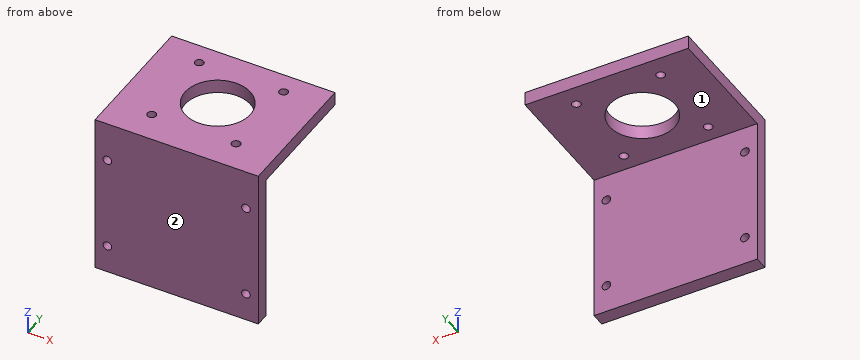
from build123d import *

# Parameters (mm, degrees)
EXTRUDE_1_DEPTH = 60
HOLE_WIZARD_2_D = 24
HOLE_WIZARD_3_D = 3.2
HOLE_WIZARD_4_D = 3.2


with BuildPart() as part:
    # 草图1 → 凸台-拉伸1 (new body)
    with BuildSketch(Plane(origin=(0, 0, 0), x_dir=(0, 0, -1), z_dir=(1, 0, 0))):
        Polygon((0, 0), (0, 50), (5, 50), (5, 5), (60, 5), (60, 0), align=None)
    extrude(amount=EXTRUDE_1_DEPTH)

    # 孔2 (through all)
    with Locations(Plane.XY):
        with Locations((30, 26.75)):
            Hole(HOLE_WIZARD_2_D / 2)

    # 孔3 (through all)
    with Locations(Plane.XY):
        with Locations((14.5, 42.25), (45.5, 42.25), (45.5, 11.25), (14.5, 11.25)):
            Hole(HOLE_WIZARD_3_D / 2)

    # 孔4 (through all)
    with Locations(Plane(origin=(0, 5, 0), x_dir=(1, 0, 0), z_dir=(0, 1, 0))):
        with Locations((55.459259259, 14.749042146), (55.459259259, 49.557471264), (4.540740741, 14.749042146), (4.540740741, 49.557471264)):
            Hole(HOLE_WIZARD_4_D / 2)


solid = part.part
Build history of the part. All positions in model axes, mm. Face numbers are marked on the shaded views. A direction names the side the tool comes from. Round coordinates to 2 decimals unless told otherwise and drop trailing zeros. Write each loop counter-clockwise with the first axis right and the second up, starting at its lowest first coordinate (ties: lowest second). Pieces come first, ordered by that corner, then holes. Notation, with made-up numbers: M 53.5,-30 L 77.5,-30 A10 ccw 77.5,-24 Z; hole C -23,-37.75 d4. An arc over 180 degrees is marked long. Answer as a JSON object with one key per item and string values. Group by question number.
(1) Cut at D-D (y = 42.25). Give the cut face in (x, z).
(2) Cut at B-B (y = 26.75). Give the cut face in (x, z), and give its area (3 significant figures).
(3) Which spindle directions (+Z, -Z, +X, -X, +Y, -Y) get a long thin tool onto all of the face, cutting with end or side? Do the marked faces 1 and 2. Say none if no direction does.
(4) Cut at A-A (x = 45.5). Give the cut face in (y, z), and give its area (3 significant figures).
(5) Drill centre lines: L1, parallel to X at y = 42, z = -3; L2, parallel to Y at x = 30, z = -2; L3, parallel to Z at x = 44, y = 46.5. Where is each one in solid material? Low to high.
(6) Cut at C-C (x = 30). Give the cut face in (y, z).
(7) Flat gauge pins, fed straight in: pin 1 (2.5 mm diameter, centred on x = 45.5, y = 11.25, fed in from +Z); pin 2 (5 mm diameter, centred on x = 14.5, y = 42.25, fed in from -Z); pin 3 (16.5 mm diameter, centred on x = 18.5, z = -45.5, fed in from +Y). Where does each tip first touch, or does it go through?
Responses:
{
 "1": {"outline": "M 0,-5 L 12.9,-5 L 12.9,0 L 0,0 Z; M 16.1,-5 L 43.9,-5 L 43.9,0 L 16.1,0 Z; M 47.1,-5 L 60,-5 L 60,0 L 47.1,0 Z"},
 "2": {"outline": "M 0,-5 L 18,-5 L 18,0 L 0,0 Z; M 42,-5 L 60,-5 L 60,0 L 42,0 Z", "area": "180 mm2"},
 "3": {"face 1": "-Z, +X, -X, +Y", "face 2": "+Z, -Z, +X, -X, -Y"},
 "4": {"outline": "M 0,-60 L 5,-60 L 5,-5 L 9.65,-5 L 9.65,0 L 0,0 Z; M 12.85,-5 L 40.65,-5 L 40.65,0 L 12.85,0 Z; M 43.85,-5 L 50,-5 L 50,0 L 43.85,0 Z", "area": "493 mm2"},
 "5": {"L1": "x = 0 to 12.92, 16.08 to 43.92, 47.08 to 60", "L2": "y = 0 to 14.75, 38.75 to 50", "L3": "z = -5 to 0"},
 "6": {"outline": "M 0,-60 L 5,-60 L 5,-5 L 14.75,-5 L 14.75,0 L 0,0 Z; M 38.75,-5 L 50,-5 L 50,0 L 38.75,0 Z"},
 "7": {"pin 1": "passes through", "pin 2": "stops at z = -5", "pin 3": "stops at y = 5"}
}
